CAD build for the part. Positions are in the model's coordinates, mm. A direction names the side the tool comes from. Round coordinates to 2 decimals unless told otherwise and drop trailing zeros. Write each loop counter-clockwise with the first axis right and the second up, starting at its lowest first coordinate (ties: lowest second). Pieces come first, ordered by that corner, then holes. Notation, with made-up numbers: (-38.75, 79.5) - (-24.75, 79.5) arc R18 cw to (-24.75, 111.5) - close; hole circle Ø1 at (16, -14.5). An arc over 180 degrees is marked (long way). Answer in a Markdown table with one row per item.
```python
from build123d import *

# Parameters (mm, degrees)
CHAMFER2_SIZE = 2.54


with BuildPart() as part:
    # Sketch1 → Revolve-Thin2 (revolve)
    with BuildSketch(Plane.XY, mode=Mode.PRIVATE) as revolve_thin2_sk:
        Polygon((16.254988293, 6.35), (27.94, 9.480989451), (27.94, 15.24), (-2.54, 15.24), (-2.54, -2.54), (27.94, -2.54), (27.94, 3.219010549), align=None)
        with BuildLine():
            Line((15.597587918, 8.803451599), (25.4, 11.43))
            Line((25.4, 11.43), (25.4, 12.7))
            Line((25.4, 12.7), (0, 12.7))
            Line((0, 12.7), (0, 0))
            Line((0, 0), (25.4, 0))
            Line((25.4, 0), (25.4, 1.27))
            Line((25.4, 1.27), (15.597587918, 3.896548401))
            ThreePointArc((15.597587918, 3.896548401), (13.714988293, 6.35), (15.597587918, 8.803451599))
        make_face(mode=Mode.SUBTRACT)
    revolve(revolve_thin2_sk.sketch.rotate(Axis((-16.51, 12.7, 0), (0, -1, 0)), 90), axis=Axis((-16.51, 12.7, 0), (0, -1, 0)))

    # Chamfer2
    chamfer2_edges = [part.edges().sort_by_distance(p)[0] for p in [
        (-16.51, -2.54, -13.97),
        (-16.51, 15.24, -13.97),
        (-16.51, 15.24, -44.45),
    ]]
    chamfer(chamfer2_edges, length=CHAMFER2_SIZE)


solid = part.part
```
Q1. Saw through at C-C on y = 5.25. List the corners of the cut face in (x, z), then the cut area to 3 significant figures.
Computed:
| item | result |
|---|---|
| outline | circle Ø73.74 at (-16.51, 0); circle Ø33.02 at (-16.51, 0); hole circle Ø60.95 at (-16.51, 0); hole circle Ø27.94 at (-16.51, 0) |
| area | 1,600 mm2 |
Q2. 3-axis set-ups, long thin cutter, end or side, ignore diameter. For faces 5 (the cylindrical face through (-46.551, 11.113, -32.761)), 6 (the conical face through (-26.571, 6.546, 31.949)): which of +Z, -Z, +X, -X, +Y, -Y reach the whole face in a straight line?
Computed:
| item | result |
|---|---|
| face 5 | +Y, -Y |
| face 6 | none |
Q3. Flat gauge pins, fed straight in: pin 1 (10 mm diameter, centred on y = 10, z = -12.5, fed in from +X); pin 2 (1.5 mm diameter, centred on y = 11.5, z = -0.5, fed in from +X); pin 3 (10 mm diameter, centred on x = 1, y = 1, fed in from -Z). Where does each tip first touch, or does it go through?
Computed:
| item | result |
|---|---|
| pin 1 | stops at x = 27.3 |
| pin 2 | stops at x = 27.94 |
| pin 3 | stops at z = -42.65 |
Q4. Saw through at A-A on z = 9. Count the separate pieces of the cut face and the enclosed holes in it, then the cut area to 3 significant figures.
Computed:
| item | result |
|---|---|
| separate pieces | 2 |
| enclosed holes | 2 |
| area | 548 mm2 |
Q5. Pull direction X, two halves, no side cores. Call faces 1 (the conical face through (20.8, 15.1, 19.4)), 2 (the conical face through (15.3, 3.77, -7.06)), 3 (the flat face through (-17, -2.54, -19)), 4 (the conical face through (-26.34, 8.97, 31.21)): released by +X, released by -X, zero draft, split by the parting line, or undercut.
Computed:
| item | result |
|---|---|
| face 1 | split by the parting line |
| face 2 | undercut |
| face 3 | zero draft |
| face 4 | undercut |
Q6. Drill centre lines: line 1 (X direction, y = 12.1, z = 0); line 2 (Z direction, x = -28.5, y = 1); line 3 (Y direction, x = 2, z = 12). Where is each one in solid material? Low to high.
Computed:
| item | result |
|---|---|
| line 1 | x = -60.96 to -58.42, -33.02 to -30.48, -2.54 to 0, 25.4 to 27.94 |
| line 2 | z = -42.8 to -40.16, -11.35 to -7.17, 7.17 to 11.35, 40.16 to 42.8 |
| line 3 | y = -2.54 to 0, 12.7 to 15.24 |
